The figure shows three views and two pictorial views of one solid part (mm, origin at its lowest corner). Answer the questions. Round coordinates to 2 decimals unless told otherwise and drop trailing zeros. Write each loop counter-clockwise with the first axis right and the second up, starting at its lowest first coordinate (ties: lowest second). Pieces come first, ordered by that corner, then holes. Notation, with made-up numbers: (71, 47.25) -> (105, 47.25) arc R21 ccw to (105, 60.25) -> close; hole circle Ø4 at (32.5, 7.5). An arc over 180 degrees is marked (long way). One line per item, written item: value.
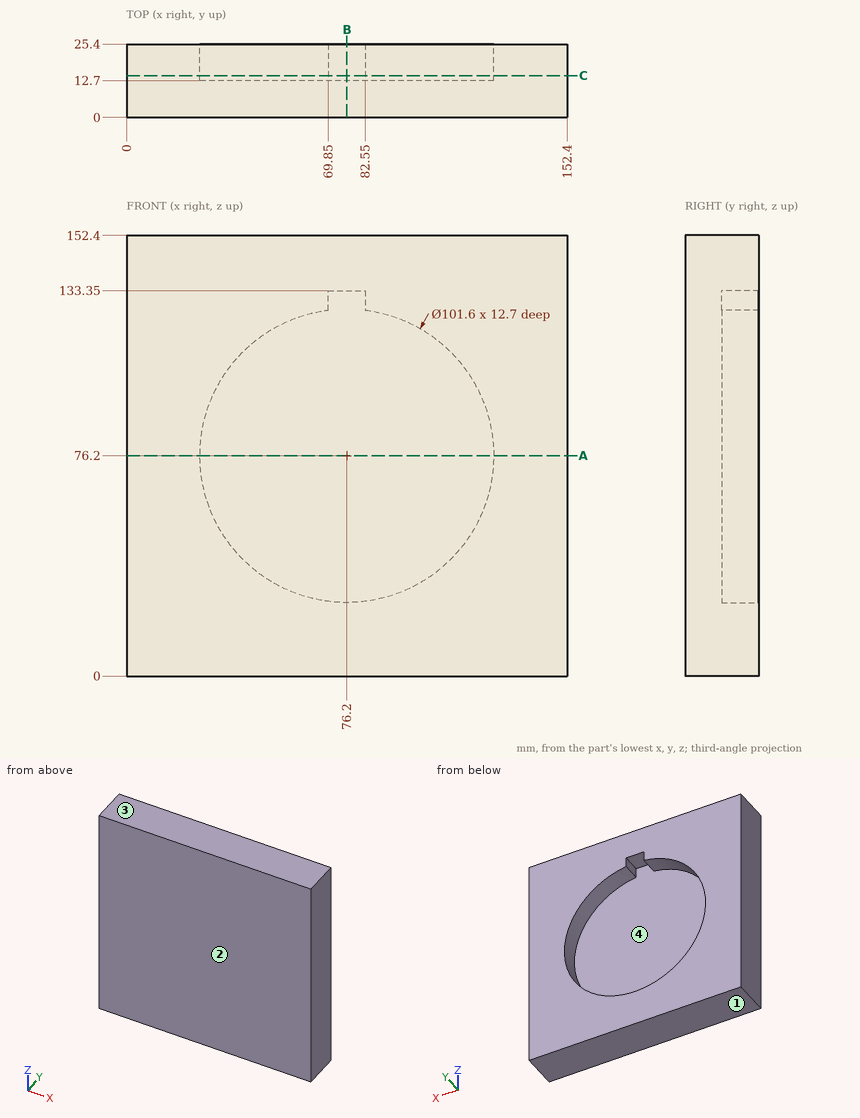
(1) Consider probe 1 along X at (y, z) = (21.75, 76.2); probe 2 along Z at (x, y) = (76.2, 21); probe 3 along Y at (x, z) = (43, 78). Determine where each line is inside the solid, lowest interval first.
Reported:
probe 1: x = 0 to 25.4, 127 to 152.4
probe 2: z = 0 to 25.4, 133.35 to 152.4
probe 3: y = 0 to 12.7
(2) For a pull along Z with two mould halves and no side action, classify the marked faces 1, 2, 3 and 4 as pulls with the +Z half, pulls with the -Z half, needs draft (parallel to the pull), parting line crosses it, or undercut.
Reported:
face 1: pulls with the -Z half
face 2: needs draft
face 3: pulls with the +Z half
face 4: undercut
(3) Find section B-B on x = 76.2. Give the vertices of the cut face in (y, z), plus the area to 3 significant figures.
Reported:
outline: (0, 0) -> (25.4, 0) -> (25.4, 25.4) -> (12.7, 25.4) -> (12.7, 133.35) -> (25.4, 133.35) -> (25.4, 152.4) -> (0, 152.4) -> close
area: 2,500 mm2
(4) A flat-ended cylindrical pin translates along its axis: pin 1 Ø12 at (x, z) = (95.5, 64) entering from +Y. Find the tip coordinate at first contact, or state that the pin passes through.
Reported:
pin 1: stops at y = 12.7
(5) Find section C-C on y = 14.5. Give the vertices of the cut face in (x, z), plus the area to 3 significant figures.
Reported:
outline: (0, 0) -> (152.4, 0) -> (152.4, 152.4) -> (0, 152.4) -> close; hole (69.85, 126.6) arc R50.8 ccw (long way) to (82.55, 126.6) -> (82.55, 133.35) -> (69.85, 133.35) -> close
area: 15,000 mm2
(6) Find section A-A on z = 76.2. Give the vertices of the cut face in (x, y).
Reported:
outline: (0, 0) -> (152.4, 0) -> (152.4, 25.4) -> (127, 25.4) -> (127, 12.7) -> (25.4, 12.7) -> (25.4, 25.4) -> (0, 25.4) -> close
